Geometry check sheet. Reference: drawing and pictorial views, mm from the part's lowest x, y, z. Round coordinates to 2 decimals unless told otherwise and drop trailing zeros. Order: outer loops, then holes, each group sorted by start corner. A loop starts at its lowest first (then second) coordinate and runs counter-clockwise, first axis right, second up.
(1) Thickness scan on L1, parallel to X at y = 10.25, z = 4.5; L2, parallel to Y at x = 36, z = 7.5; L3, parallel to X at y = 9.25, z = 2.25. Record the ranges inside material, lowest first.
(2) Cross-section at C-C on x = 57.5. Enter the section's corners in (y, z).
(3) Gauge pin test, flat ends, axial feed: P1, Ø4.5, axis at x = 17.5, z = 3, coming from the +Y side; P2, Ø1.5, axis at x = 55, y = 10, coming from the -Z side. Record the tip position at first contact, or that the pin passes through.
(4) Cross-section at D-D on x = 14. Enter the section's corners in (y, z).
(5) Draft check along X on the marked faces 1, 2 and 3. Enter one of: pulls with the +X half, pulls with the -X half, needs draft (parallel to the pull), parting line crosses it, or undercut.
(6) Cross-section at A-A on z = 4.5. Enter the section's corners in (x, y).
(7) Cross-section at B-B on y = 10.5. Enter the section's corners in (x, z), and give its area (3 significant figures).
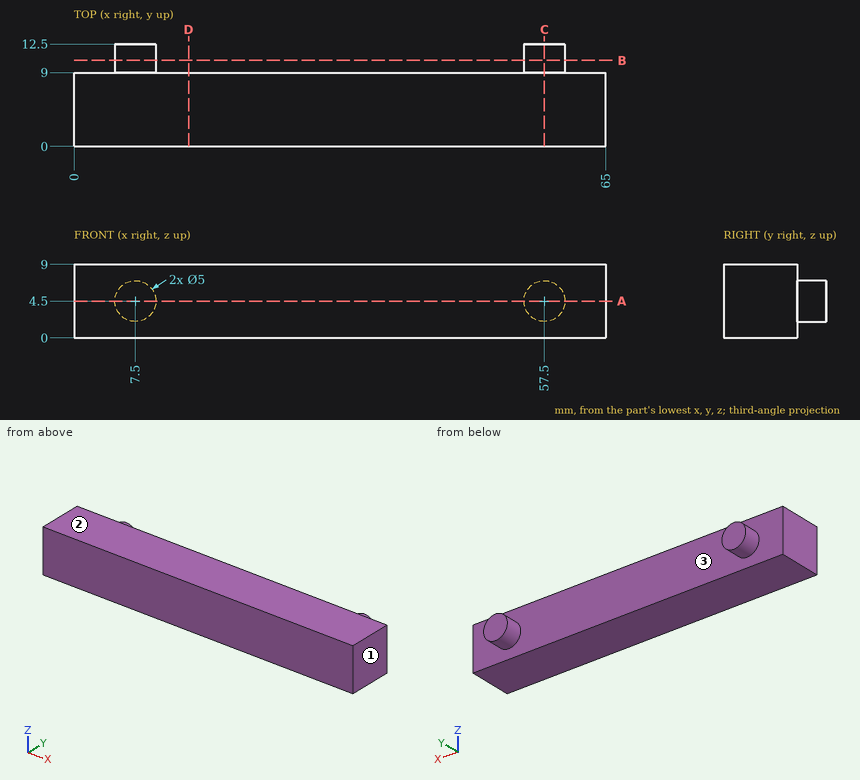
Found:
1. L1: x = 5 to 10, 55 to 60
1. L2: y = 0 to 9
1. L3: x = 6.41 to 8.59, 56.41 to 58.59
2. outline: (0, 0) - (9, 0) - (9, 2) - (12.5, 2) - (12.5, 7) - (9, 7) - (9, 9) - (0, 9) - close
3. P1: stops at y = 9
3. P2: stops at z = 2.71
4. outline: (0, 0) - (9, 0) - (9, 9) - (0, 9) - close
5. face 1: pulls with the +X half
5. face 2: needs draft
5. face 3: undercut
6. outline: (0, 0) - (65, 0) - (65, 9) - (60, 9) - (60, 12.5) - (55, 12.5) - (55, 9) - (10, 9) - (10, 12.5) - (5, 12.5) - (5, 9) - (0, 9) - close
7. outline: circle Ø5 at (7.5, 4.5); circle Ø5 at (57.5, 4.5)
7. area: 39.3 mm2
